```python
from build123d import *

# Parameters (mm, degrees)
EXTRUDE_1_DEPTH                 = 206
SKETCH_2_W                      = 252
SKETCH_2_H                      = 252
CUT_EXTRUDE_1_DEPTH             = 123.6
SKETCH_3_W                      = 210
SKETCH_3_H                      = 210
CUT_EXTRUDE_2_DEPTH             = 144.2
SHELL_1_T                       = -5
SKETCH_4_R                      = 50
CUT_EXTRUDE_3_DEPTH             = 455.80065963
EXTRUDE_2_DEPTH                 = 10
PATTERN_CIRCULAR_1_COUNT        = 4
PATTERN_CIRCULAR_1_COPY_1_DEPTH = 10
PATTERN_CIRCULAR_1_COPY_2_DEPTH = 10
PATTERN_CIRCULAR_1_COPY_3_DEPTH = 10


with BuildPart() as part:
    # 草图1 → 凸台-拉伸1 (new body)
    with BuildSketch(Plane.XY):
        Polygon((-305, 183), (-183, 305), (183, 305), (305, 183), (305, -183), (183, -305), (-183, -305), (-305, -183), align=None)
    extrude(amount=EXTRUDE_1_DEPTH)

    # 草图2 → 切除-拉伸1 (cut)
    with BuildSketch(Plane.XY.offset(206)):
        Rectangle(SKETCH_2_W, SKETCH_2_H)
    extrude(amount=-CUT_EXTRUDE_1_DEPTH, mode=Mode.SUBTRACT)

    # 草图3 → 切除-拉伸2 (cut)
    with BuildSketch(Plane.XY.offset(206)):
        Rectangle(SKETCH_3_W, SKETCH_3_H)
    extrude(amount=-CUT_EXTRUDE_2_DEPTH, mode=Mode.SUBTRACT)

    # 抽壳1
    shell_1_openings = [part.faces().sort_by_distance(p)[0] for p in [
        (0, 0, 0),
    ]]
    offset(amount=SHELL_1_T, openings=shell_1_openings, kind=Kind.INTERSECTION)

    # 草图4 → 切除-拉伸3 (cut, through all)
    with BuildSketch(Plane.XY.offset(61.8)):
        Circle(SKETCH_4_R)
    extrude(amount=-CUT_EXTRUDE_3_DEPTH, mode=Mode.SUBTRACT)

    # 草图5 → 凸台-拉伸2 (add)
    with BuildSketch(Plane(origin=(0, 91.5, 0), x_dir=(1, 0, 0), z_dir=(0, 1, 0))):
        Polygon((-131, -82.4), (-300, -112.19925974), (-300, -200.864779471), (-131, -200.864779471), align=None)
    extrude_2 = extrude(amount=-EXTRUDE_2_DEPTH)

    # 镜向1: 凸台-拉伸2 across plane
    add(extrude_2.mirror(Plane.ZX))

    # 阵列(圆周)1: 凸台-拉伸2 ×4 about axis
    pattern_circular_1_axis = Axis((0, 0, 0), (0, 0, 1))
    for i in range(1, PATTERN_CIRCULAR_1_COUNT):
        add(extrude_2.rotate(pattern_circular_1_axis, i * 360 / PATTERN_CIRCULAR_1_COUNT))

    # 阵列(圆周)1 copy 1 sketch → 阵列(圆周)1 copy 1 (add)
    with BuildSketch(Plane.YZ.offset(91.5)):
        Polygon((-131, 82.4), (-300, 112.19925974), (-300, 200.864779471), (-131, 200.864779471), align=None)
    extrude(amount=-PATTERN_CIRCULAR_1_COPY_1_DEPTH)

    # 阵列(圆周)1 copy 2 sketch → 阵列(圆周)1 copy 2 (add)
    with BuildSketch(Plane(origin=(0, 91.5, 0), x_dir=(-1, 0, 0), z_dir=(0, 1, 0))):
        Polygon((-131, 82.4), (-300, 112.19925974), (-300, 200.864779471), (-131, 200.864779471), align=None)
    extrude(amount=-PATTERN_CIRCULAR_1_COPY_2_DEPTH)

    # 阵列(圆周)1 copy 3 sketch → 阵列(圆周)1 copy 3 (add)
    with BuildSketch(Plane(origin=(-91.5, 0, 0), x_dir=(0, -1, 0), z_dir=(-1, 0, 0))):
        Polygon((-131, 82.4), (-300, 112.19925974), (-300, 200.864779471), (-131, 200.864779471), align=None)
    extrude(amount=-PATTERN_CIRCULAR_1_COPY_3_DEPTH)


solid = part.part
```
Verification items for the finished model (mm, model axes). A direction names the side the tool comes from. Coordinates: 2 decimals unless noted, no trailing zeros. Write each loop counter-clockwise with the first axis right and the second up, starting at its lowest first coordinate (ties: lowest second). Pieces come first, ordered by that corner, then holes. Notation, with made-up numbers: (-21.5, 45) - (18.5, 45) arc R28 cw to (18.5, 78) - close; hole circle Ø7 at (79.5, 82.5). An arc over 180 degrees is marked (long way). One line per question, with ' | ' between items. Start each with the question number.
1. Access from +Z, -Z, +X, -X, +Y, -Y to the whole of each face (thin tool, end or side, straight path). Record for faces 4 (the flat face through (-214.32, -86.57, 97.09)), 5 (the flat face through (105, -1, 72)).
2. Draft check along X on faces 1 (the flat face through (126, -2, 145)), 2 (the flat face through (86.57, 214.32, 97.09)), 3 (the flat face through (305, 3, 102)). Enter one of: released by +X, released by -X, zero draft, split by the parting line, or undercut.
3. Gauge pin test, flat ends, axial feed: P1, Ø12, axis at y = -222, z = 114, coming from the -X side; P2, Ø4, axis at x = -40, y = -226, coming from the -Z side; P3, Ø1, axis at y = -217, z = 104.5, coming from the -X side. Record the tip position at first contact, or that the pin passes through.
4. Material ranges on line 1 along Y through (x, z) = (-35, 104); line 2 along Y through (x, z) = (0, 58.55), recorded low to high.
5. Section check A-A (y = 0). Enter the section's corners in (x, z), plus the area to 3 significant figures.
6. Section check C-C (y = 215). Enter the section's corners in (x, z).
7. Section check D-D (z = 144.5). Count the separate pieces of the cut face and the enclosed holes in it, plus the area to 3 significant figures.
Computed values:
1) face 4: -Z | face 5: +Z
2) face 1: undercut | face 2: undercut | face 3: released by +X
3) P1: x = -272 | P2: z = 201 | P3: x = -271.5
4) line 1: -305 to -300, -131 to -126, 126 to 131, 300 to 305 | line 2: -305 to -300, -110 to -50, 50 to 110, 300 to 305
5) outline: (-305, 0) - (-300, 0) - (-300, 201) - (-131, 201) - (-131, 77.4) - (-110, 77.4) - (-110, 56.8) - (-50, 56.8) - (-50, 61.8) - (-105, 61.8) - (-105, 82.4) - (-126, 82.4) - (-126, 206) - (-305, 206) - close; (50, 56.8) - (110, 56.8) - (110, 77.4) - (131, 77.4) - (131, 201) - (300, 201) - (300, 0) - (305, 0) - (305, 206) - (126, 206) - (126, 82.4) - (105, 82.4) - (105, 61.8) - (50, 61.8) - close | area: 6,000 mm²
6) outline: (-273, 0) - (-265.93, 0) - (-265.93, 201) - (265.93, 201) - (265.93, 0) - (273, 0) - (273, 206) - (-273, 206) - close; (-91.5, 97.21) - (-81.5, 97.21) - (-81.5, 200.86) - (-91.5, 200.86) - close; (81.5, 97.21) - (91.5, 97.21) - (91.5, 200.86) - (81.5, 200.86) - close
7) separate pieces: 1 | enclosed holes: 9 | area: 29,300 mm²
